```python
from build123d import *

# Parameters (mm, degrees)
F0_R      = 31.223387
F1_DEPTH  = 25.4
F2_R      = 8.233422
F3_DEPTH  = 25.4
F3_FACE_R = 8.233422
F4_DEPTH  = 25.4


with BuildPart() as f1:
    # F0 (on Front) → F1 (new body)
    with BuildSketch(Plane.XZ):
        Circle(F0_R)
    extrude(amount=F1_DEPTH)

    # F2 (on face) → F3 (join)
    with BuildSketch(Plane.XZ.offset(25.4)):
        Circle(F2_R)
    extrude(amount=F3_DEPTH)

    # F3_face (on face) → F4 (join)
    with BuildSketch(Plane.XZ.offset(50.8)):
        Circle(F3_FACE_R)
    extrude(amount=-F4_DEPTH)


solid = f1.part
```
Here's how the part is built. I have some questions about the finished solid (model axes, mm). A direction names the side the tool comes from. Coordinates: 2 decimals unless noted, no trailing zeros. Order: outer loops, then holes, each group sorted by start corner. A loop starts at its lowest first (then second) coordinate and runs counter-clockwise, first axis right, second up. Notation, with made-up numbers: M 17.5,36.5 L 23.5,36.5 A17 cw 23.5,42.5 Z; hole C 39,19 d4. An arc over 180 degrees is marked long. Answer as a JSON object with one key per item and string values. Group by question number.
(1) Suppose I cut it at B-B, the plane z = 0. Please give me the cut outline in (x, y).
(2) Suppose I cut it at D-D, the plane z = -20. Please give me the cut outline in (x, y), then the cut area to 3 significant figures.
(3) Suppose I cut it at A-A, the plane x = 0. Please give me the cut outline in (y, z).
(4) Suppose I cut it at C-C, the plane y = -3.5. Please give me the cut outline in (x, z).
(5) I need wall thicknesses on probe 1 along Y at (x, z) = (-9, 2); probe 2 along X at (y, z) = (-19, -2.5); probe 3 along X at (y, z) = (-3, -4.5). Which ranges of each line are inside material? Lowest first, please.
(6) For pin 1 (1 mm diameter, centred on x = 4, y = -9.5, fed in from -Z); pin 2 (5 mm diameter, centred on x = -1.5, z = 12.5, fed in from -Y); pin 3 (5 mm diameter, centred on y = -21, z = -20.5, fed in from -X), each with a flat end and sliding along its axis, tell me the tip position at first contact or that it passes through.
(7) Which directions (+Z, -Z, +X, -X, +Y, -Y) give clear straight access to the entire face, cutting with the end or side of a thin tool? Please do faces 1 (the face through (0, 0, 0)), 2 (the face through (7, -25.4, -7)).
Values found:
{
 "1": {"outline": "M -31.22,-25.4 L -8.23,-25.4 L -8.23,-50.8 L 8.23,-50.8 L 8.23,-25.4 L 31.22,-25.4 L 31.22,0 L -31.22,0 Z"},
 "2": {"outline": "M -23.98,-25.4 L 23.98,-25.4 L 23.98,0 L -23.98,0 Z", "area": "1,220 mm^2"},
 "3": {"outline": "M -50.8,-8.23 L -25.4,-8.23 L -25.4,-31.22 L 0,-31.22 L 0,31.22 L -25.4,31.22 L -25.4,8.23 L -50.8,8.23 Z"},
 "4": {"outline": "C 0,0 d62.45"},
 "5": {"probe 1": "y = -25.4 to 0", "probe 2": "x = -31.12 to 31.12", "probe 3": "x = -30.9 to 30.9"},
 "6": {"pin 1": "stops at z = -31.03", "pin 2": "stops at y = -25.4", "pin 3": "stops at x = -25.51"},
 "7": {"face 1": "+Z, -Z, +X, -X, +Y", "face 2": "-Y"}
}
